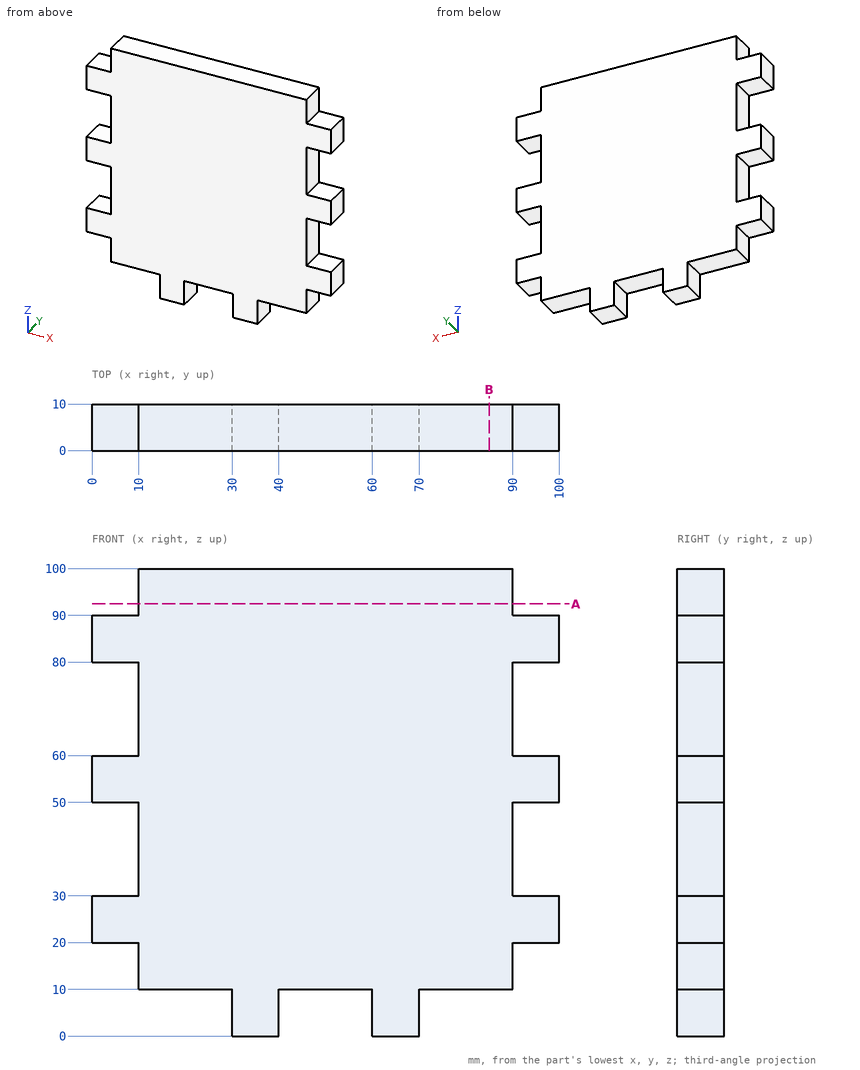
Input: dimensioned drawing with shaded views. Units: mm. Origin: part minimum x, y, z. Round coordinates to 2 decimals unless told otherwise and drop trailing zeros. Order: outer loops, then holes, each group sorted by start corner. A loop starts at its lowest first (then second) coordinate and runs counter-clockwise, first axis right, second up. Notation, with made-up numbers: (-38.75, 59.5) -> (-31.75, 59.5) arc R25 cw to (-31.75, 79.5) -> close; hole circle Ø5 at (-33, 8). An arc over 180 degrees is marked (long way). One line per item, written item: value. Start each with the question number.
Q1. Section query A-A (z = 92.5). Return the cut outline in (x, y), plus the area to 3 significant figures.
Q2. Pin query (flat end, axial travel): pin 1 (3 mm diameter, centred on x = 96, y = 5, fed in from +Z); pin 2 (3 mm diameter, centred on y = 6, z = 95, fed in from +X); pin 3 (3 mm diameter, centred on y = 3, z = 36.5, fed in from -X); pin 4 (2 mm diameter, centred on x = 14.5, z = 50.5, fed in from -Y). Return the tip coordinate at first contact, or that it passes through.
Q3. Material intervals for probe 1 along Z at (x, y) = (8, 9); probe 2 along X at (y, z) = (3.5, 47.5); probe 3 along Z at (x, y) = (86.5, 1.25), sorted ascending.
Q4. Section query B-B (x = 85). Return the cut outline in (y, z).
Findings below:
1. outline: (10, 0) -> (90, 0) -> (90, 10) -> (10, 10) -> close
1. area: 800 mm²
2. pin 1: z = 90
2. pin 2: x = 90
2. pin 3: x = 10
2. pin 4: y = 0
3. probe 1: 20 to 30, 50 to 60, 80 to 90
3. probe 2: 10 to 90
3. probe 3: 10 to 100
4. outline: (0, 10) -> (10, 10) -> (10, 100) -> (0, 100) -> close
